Autodesk Inventor part; units mm, degrees
ref_plane "Work Plane1" through (-10.3839, 4.1, 4.0025) normal (0, 1, 0) x (0, 0, 1)
ref_plane "YZ Plane" through (0, 0, 0) normal (1, 0, 0) x (0, 1, 0)
ref_plane "XZ Plane" through (0, 0, 0) normal (0, 1, 0) x (-1, 0, 0)
sketch "Sketch1" plane through (0, 0, 0) normal (0, 1, 0) x (-1, 0, 0)
  line L0 (4.4839, 27.6452) -> (-35.5161, 27.6452)
  line L1 (-35.5161, 27.6452) -> (-35.5161, -32.3548)
  line L2 (-35.5161, -32.3548) -> (4.4839, -32.3548)
  line L3 (4.4839, -32.3548) -> (4.4839, 27.6452)
  point P0 (0, 0)
  dimension "d0" = 60
  dimension "d1" = 40
extrude "Extrusion1" add sketch "Sketch1" along normal blind 5.2
fillet "Fillet1" radius 5 2 edges at (35.5161, 2.6, -32.3548) (35.5161, 2.6, 27.6452)
sketch "Sketch2" plane through (0, 0, 0) normal (0, -1, 0) x (1, 0, 0)
  circle A0 centre (30.5161, 21.6452) radius 1.5
  circle A1 centre (1.0161, 24.6452) radius 1.5
  circle A2 centre (1.0161, -29.3548) radius 1.5
  circle A3 centre (30.5161, -26.3548) radius 1.5
  point P0 (0, 0)
hole "Hole1" at (30.5161, 0, 21.6452) at (30.5161, 0, -26.3548) at (1.0161, 0, -29.3548) at (1.0161, 0, 24.6452) direction (0, 1, 0) diameter 3 end through all
sketch "Sketch3" plane through (0, 5.2, 0) normal (0, 1, 0) x (1, 0, 0)
  circle A0 centre (-2.4839, -11.6452) radius 7.9
  point P0 (0, 0)
ref_plane "Work Plane1" through (-10.3839, 4.1, 4.0025) normal (0, 1, 0) x (0, 0, 1)
extrude "Extrusion2" cut sketch "Sketch3" against normal up to surface (1.1 mm away)
sketch "Sketch4" plane through (-2.4839, 4.1, 11.6452) normal (0, 1, 0) x (1, 0, 0)
  arc A0 (-2, 5.3376) -> (-2, -5.3376) centre (0, 0) ccw
  circle A1 centre (0, 0) radius 5.5
  circle A2 centre (0, 0) radius 5.7
  point P0 (2.4839, 11.6452)
  dimension "d14" = 11.4
extrude "Extrusion3" cut sketch "Sketch4" against normal through all contours A2 A0 | A1
sketch "Sketch5" plane through (0, 0, 0) normal (0, -1, 0) x (1, 0, 0)
  circle A0 centre (24.0161, 11.1452) radius 6
  circle A1 centre (24.0161, -15.8548) radius 6
  line L0 (24.0161, 11.1452) -> (24.0161, -15.8548) construction
  line L1 (18.0161, 11.1452) -> (18.0161, -15.8548)
  line L2 (30.0161, -15.8548) -> (30.0161, 11.1452)
  arc A2 (30.0161, 11.1452) -> (18.0161, 11.1452) centre (24.0161, 11.1452) ccw
  arc A3 (18.0161, -15.8548) -> (30.0161, -15.8548) centre (24.0161, -15.8548) ccw
  point P0 (0, 0)
  point P1 (24.0161, -2.3548)
extrude "Extrusion4" cut sketch "Sketch5" against normal through all
properties part number "Carro XY_trava_B" material "ABS Plastic"
Read the model definition and answer for the solid it produces. Units are mm, in the model's axes. A direction names the side the tool comes from. Give positions to 0.01 mm unless a question says otherwise; leave off trailing zeros. Loops run counter-clockwise (first coordinate to the right, second up) from the corner with the lowest first, then second, coordinate; pieces in that order, holes last. Notation, with made-up numbers: M -11,50 L 31,50 A23 ccw 31,64 Z; hole C 39.25,86.5 d5. An arc over 180 degrees is marked long. Write each question's results on one line, items separated by ' | '.
1. Given pin 1 (5 mm diameter, centred on x = 7.5, z = -15, fed in from -Y), flat-ended and moving along its own axis, determine where the tip first touches the part or whether it passes through.
Values:
pin 1: stops at y = 0
2. The mould has two halves that part along Z. Classify faces 4 (the face through (34.09, 2.64, -30.85)), 5 (the face through (29.03, 2.64, 21.84)), 6 (the face through (16, 0, -2)): pulls with the +Z half, pulls with the -Z half, needs draft (parallel to the pull), parting line crosses it, or undercut.
Values:
face 4: pulls with the -Z half | face 5: undercut | face 6: needs draft
3. Section C-C on y = 1.25 is taken. Give the vertices of the cut face in (x, z).
Values:
outline: M -4.48,-32.35 L 30.52,-32.35 A5 ccw 35.52,-27.35 L 35.52,22.65 A5 ccw 30.52,27.65 L -4.48,27.65 L -4.48,16.98 A5.7 cw long -4.48,6.31 Z; hole C 1.02,-29.35 d3; hole C 1.02,24.65 d3; hole M 18.02,-15.85 A6 ccw 30.02,-15.85 L 30.02,11.15 A6 ccw 18.02,11.15 Z; hole C 30.52,-26.35 d3; hole C 30.52,21.65 d3
4. Straight lines are drawn through the part: line 1 (X direction, y = 1.8, z = -12); line 2 (Z direction, x = 0, y = 4.5); line 3 (X direction, y = 0.45, z = 21.5). For each, find the intervals that lie inside material, in ascending order. Write a range as [from, to].
Values:
line 1: x = [-4.48, 18.02], [30.02, 35.52] | line 2: z = [-32.35, -30.46], [-28.25, 4.15], [19.14, 23.54], [25.75, 27.65] | line 3: x = [-4.48, 29.02], [32.01, 35.52]
5. Section A-A on z = 1 is taken. Give the vertices of the cut face in (x, y).
Values:
outline: M -4.48,0 L 18.02,0 L 18.02,5.2 L -4.48,5.2 Z; M 30.02,0 L 35.52,0 L 35.52,5.2 L 30.02,5.2 Z
6. A tool of negligible diameter and unlimited length cuts with its end or side. For faces 1 (the face through (-4.484, 3, -13)), 2 (the face through (5.414, 4.658, 11.847)), 3 (the face through (24.148, 2.564, 17.144)), from which of +Z, -Z, +X, -X, +Y, -Y can it reach the whole face along a straight path? Write none if from no direction.
Values:
face 1: +Z, -Z, -X, +Y, -Y | face 2: +Y | face 3: +Y, -Y
7. Section B-B on x = 27 is taken. Give the vertices of the cut face in (y, z).
Values:
outline: M 0,-32.35 L 5.2,-32.35 L 5.2,-21.06 L 0,-21.06 Z; M 0,16.35 L 5.2,16.35 L 5.2,27.65 L 0,27.65 Z
8. Section D-D on z = 9.5 is taken. Give the vertices of the cut face in (x, y).
Values:
outline: M 2.8,0 L 18.02,0 L 18.02,5.2 L 5.12,5.2 L 5.12,4.1 L 2.8,4.1 Z; M 30.02,0 L 35.52,0 L 35.52,5.2 L 30.02,5.2 Z
